Read the model definition and answer for the solid it produces. Units are mm, in the model's axes. Face numbers are marked on the shaded views. A direction names the side the tool comes from. Coordinates: 2 decimals unless noted, no trailing zeros. Write each loop counter-clockwise with the first axis right and the second up, starting at its lowest first coordinate (ties: lowest second). Pieces come first, ordered by that corner, then holes. Notation, with made-up numbers: M 1,8.25 L 17,8.25 A20 cw 17,21.25 Z; hole C 85,-9 d3. An arc over 180 degrees is marked long. Write item = value, one per line.
from build123d import *

# Parameters (mm, degrees)
SKETCH2_W                      = 516
SKETCH2_H                      = 198
SKETCH2_W_2                    = 65
SKETCH2_H_2                    = 178
SKETCH2_W_3                    = 416
BOSS_EXTRUDE2_DEPTH            = 45
DRAFT3_ANGLE                   = 20
FILLET1_R                      = 10
SKETCH2_3_W                    = 416
SKETCH2_3_H                    = 178
SKETCH2_3_W_2                  = 350
SKETCH2_3_H_2                  = 80
SKETCH2_3_W_3                  = 376
SKETCH2_3_H_3                  = 68
SKETCH2_3_W_4                  = 65
BOSS_EXTRUDE3_DEPTH            = 2
CUT_EXTRUDE1_DEPTH             = 5
SKETCH2_5_W                    = 376
SKETCH2_5_H                    = 68
BOSS_EXTRUDE4_DEPTH            = 40
SKETCH2_6_W                    = 350
SKETCH2_6_H                    = 80
BOSS_EXTRUDE5_DEPTH            = 30
CUT_EXTRUDE2_REACH             = 538.858
SKETCH4_R                      = 10
CUT_EXTRUDE2_DIRECTION_2_DEPTH = 54
SKETCH5_R                      = 7.5
CUT_EXTRUDE3_DEPTH             = 15


with BuildPart() as part:
    # Sketch2 → Boss-Extrude2 (new body)
    with BuildSketch(Plane(origin=(0, 0, 0), x_dir=(1, 0, 0), z_dir=(0, 1, 0))):
        Rectangle(SKETCH2_W, SKETCH2_H)
        with Locations((215.5, 0)):
            Rectangle(SKETCH2_W_2, SKETCH2_H_2, mode=Mode.SUBTRACT)
        with Locations((-40, 0)):
            Rectangle(SKETCH2_W_3, SKETCH2_H_2, mode=Mode.SUBTRACT)
    extrude(amount=BOSS_EXTRUDE2_DEPTH)

    # Draft3
    draft3_faces = [part.faces().sort_by_distance(p)[0] for p in [
        (0, 22.5, -99),
        (258, 22.5, 0),
        (0, 22.5, 99),
        (-258, 22.5, 0),
    ]]
    draft(draft3_faces, Plane.ZX.offset(45), DRAFT3_ANGLE)

    # Fillet1
    fillet1_edges = [part.edges().sort_by_distance(p)[0] for p in [
        (-248, 22.5, 89),
        (168, 22.5, 89),
        (168, 22.5, -89),
        (-248, 22.5, -89),
        (-266.189330271, 22.5, -107.189330271),
        (266.189330271, 22.5, -107.189330271),
        (266.189330271, 22.5, 107.189330271),
        (-266.189330271, 22.5, 107.189330271),
        (248, 22.5, 89),
        (248, 22.5, -89),
        (183, 22.5, -89),
        (183, 22.5, 89),
    ]]
    fillet(fillet1_edges, radius=FILLET1_R)

    # Sketch2<3> → Boss-Extrude3 (add)
    # profile 1 of 4: a face of its own
    with BuildSketch(Plane(origin=(0, 0, 0), x_dir=(1, 0, 0), z_dir=(0, 1, 0))):
        with Locations((-40, 0)):
            Rectangle(SKETCH2_3_W, SKETCH2_3_H)
        with Locations((-63, 44)):
            Rectangle(SKETCH2_3_W_2, SKETCH2_3_H_2, mode=Mode.SUBTRACT)
        with Locations((-50, -45)):
            Rectangle(SKETCH2_3_W_3, SKETCH2_3_H_3, mode=Mode.SUBTRACT)
    # profile 2 of 4: a face of its own
    with BuildSketch(Plane(origin=(0, 0, 0), x_dir=(1, 0, 0), z_dir=(0, 1, 0))):
        with Locations((-50, -45)):
            Rectangle(SKETCH2_3_W_3, SKETCH2_3_H_3)
    # profile 3 of 4: a face of its own
    with BuildSketch(Plane(origin=(0, 0, 0), x_dir=(1, 0, 0), z_dir=(0, 1, 0))):
        with Locations((-63, 44)):
            Rectangle(SKETCH2_3_W_2, SKETCH2_3_H_2)
    # profile 4 of 4: a face of its own
    with BuildSketch(Plane(origin=(0, 0, 0), x_dir=(1, 0, 0), z_dir=(0, 1, 0))):
        with Locations((215.5, 0)):
            Rectangle(SKETCH2_3_W_4, SKETCH2_3_H)
    extrude(amount=BOSS_EXTRUDE3_DEPTH)

    # Sketch3 → Cut-Extrude1 (cut)
    with BuildSketch(Plane(origin=(0, 45, 0), x_dir=(1, 0, 0), z_dir=(0, 1, 0))):
        with BuildLine():
            Line((171, -79), (171, 79))
            ThreePointArc((171, 79), (167.192388155, 88.192388155), (158, 92))
            Line((158, 92), (-238, 92))
            ThreePointArc((-238, 92), (-247.192388155, 88.192388155), (-251, 79))
            Line((-251, 79), (-251, -79))
            ThreePointArc((-251, -79), (-247.192388155, -88.192388155), (-238, -92))
            Line((-238, -92), (158, -92))
            ThreePointArc((158, -92), (167.192388155, -88.192388155), (171, -79))
        make_face()
        with BuildLine():
            Line((193, -92), (238, -92))
            ThreePointArc((238, -92), (247.192388155, -88.192388155), (251, -79))
            Line((251, -79), (251, 79))
            ThreePointArc((251, 79), (247.192388155, 88.192388155), (238, 92))
            Line((238, 92), (193, 92))
            ThreePointArc((193, 92), (183.807611845, 88.192388155), (180, 79))
            Line((180, 79), (180, -79))
            ThreePointArc((180, -79), (183.807611845, -88.192388155), (193, -92))
        make_face()
    extrude(amount=-CUT_EXTRUDE1_DEPTH, mode=Mode.SUBTRACT)

    # Sketch2<5> → Boss-Extrude4 (add)
    with BuildSketch(Plane(origin=(0, 0, 0), x_dir=(1, 0, 0), z_dir=(0, 1, 0))):
        with Locations((-50, -45)):
            Rectangle(SKETCH2_5_W, SKETCH2_5_H)
    extrude(amount=BOSS_EXTRUDE4_DEPTH)

    # Sketch2<6> → Boss-Extrude5 (add)
    with BuildSketch(Plane(origin=(0, 0, 0), x_dir=(1, 0, 0), z_dir=(0, 1, 0))):
        with Locations((-63, 44)):
            Rectangle(SKETCH2_6_W, SKETCH2_6_H)
    extrude(amount=BOSS_EXTRUDE5_DEPTH)

    # Cut-Extrude2: up to this face of the body (flat: up to its plane)
    cut_extrude2_end = Plane(part.part.faces().sort_by_distance((168, 21, 0))[0])
    # Sketch4 → Cut-Extrude2 (cut, up to the picked face)
    with BuildSketch(Plane.ZY.offset(-248), mode=Mode.PRIVATE) as cut_extrude2_sk1:
        with Locations((-39, 21)):
            Circle(SKETCH4_R)
    cut_extrude2_tool1 = split(extrude(cut_extrude2_sk1.sketch, amount=CUT_EXTRUDE2_REACH, mode=Mode.PRIVATE), bisect_by=cut_extrude2_end, keep=Keep.BOTH, mode=Mode.PRIVATE)
    add(cut_extrude2_tool1.solids().sort_by(Axis((248, 21, -39), (-1, 0, 0)))[0], mode=Mode.SUBTRACT)

    # Sketch4 → Cut-Extrude2 direction 2 (cut)
    with BuildSketch(Plane.ZY.offset(-248)):
        with Locations((-39, 21)):
            Circle(SKETCH4_R)
    extrude(amount=-CUT_EXTRUDE2_DIRECTION_2_DEPTH, mode=Mode.SUBTRACT)

    # Sketch5 → Cut-Extrude3 (cut)
    with BuildSketch(Plane(origin=(183, 0, 0), x_dir=(0, 0, -1), z_dir=(1, 0, 0))):
        with Locations((-29, 21)):
            Circle(SKETCH5_R)
    extrude(amount=-CUT_EXTRUDE3_DEPTH, mode=Mode.SUBTRACT)


solid = part.part
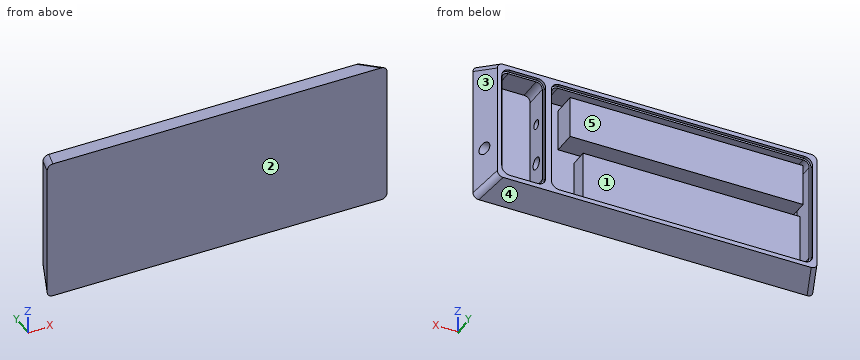
Item 1: Which of the six approach directions +Z, -Z, +X, -X, +Y, -Y give full straight-line access (tool end or side, diameter ignored) to the marked faces 1 and 2?
Worked answers:
face_1 = +Y
face_2 = +Z, -Z, +X, -X, -Y
Item 2: Find section C-C (z = -12.5). Determine the outline of the cut face in (x, y), and give its area (3 significant figures).
Worked answers:
outline = M -274.38,0 L 274.38,0 L 258,45 L 251,45 L 251,40 L 248,40 L 248,2 L 183,2 L 183,40 L 180,40 L 180,45 L 171,45 L 171,40 L 168,40 L 168,2 L 112,2 L 112,30 L -238,30 L -238,2 L -248,2 L -248,40 L -251,40 L -251,45 L -258,45 Z
area = 13,000 mm²
Item 3: Flat-ended cylindrical pins translate along their axes: pin 1 (18 mm diameter, centred on y = 21, z = -39, fed in from -X); pin 2 (11.5 mm diameter, centred on x = 30.5, y = 18, fed in from +Z); pin 3 (6 mm diameter, centred on x = 160, z = -56.5, fed in from +Y). Find the tip coordinate at first contact, or state that the pin passes through.
Worked answers:
pin_1 = -270.01
pin_2 = 110.92
pin_3 = 2
Item 4: Find section B-B (x = -173). Determine the outline of the cut face in (y, z).
Worked answers:
outline = M 0,-115.38 L 45,-99 L 45,-92 L 40,-92 L 40,-89 L 2,-89 L 2,-84 L 30,-84 L 30,-4 L 2,-4 L 2,11 L 40,11 L 40,79 L 2,79 L 2,89 L 40,89 L 40,92 L 45,92 L 45,99 L 0,115.38 Z
Item 5: Consider line 1 along Y through (x, z) = (177, 29); line 2 along Y through (x, z) = (252.5, -39); line 3 along X through (y, z) = (22.5, 83.5). Determine where each line is inside the solid, lowest interval first. Write a range as from..to.
Worked answers:
line_1 = 0..13.5, 28.5..45
line_2 = 0..11, 31..45
line_3 = -266.19..-246.93, 166.93..184.07, 246.93..266.19
Item 6: For a pull along Z with two mould halves and no side action, classify the marked faces 3, 4 and 5 as released by +Z, released by -Z, zero draft, split by the parting line, or undercut.
Worked answers:
face_3 = zero draft
face_4 = released by -Z
face_5 = undercut
Item 7: Find section A-A (z = 29). Determine the outline of the cut face in (x, y), and give its area (3 significant figures).
Worked answers:
outline = M -274.38,0 L 274.38,0 L 258,45 L 251,45 L 251,40 L 248,40 L 248,2 L 183,2 L 183,13.5 L 168,13.5 L 168,2 L 138,2 L 138,40 L -238,40 L -238,2 L -248,2 L -248,40 L -251,40 L -251,45 L -258,45 Z; M 168,28.5 L 183,28.5 L 183,40 L 180,40 L 180,45 L 171,45 L 171,40 L 168,40 Z
area = 17,300 mm²
Item 8: Find section D-D (z = -39). State how many separate pieces and enclosed holes the cut face has, and give its area (3 significant figures).
Worked answers:
separate_pieces = 3
enclosed_holes = 0
area = 12,300 mm²
